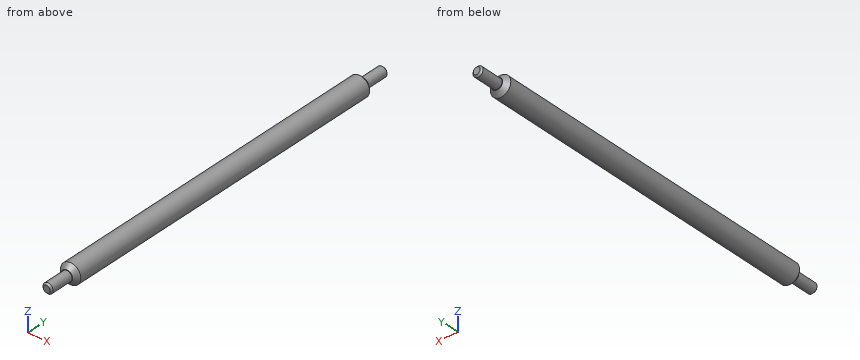
```python
from build123d import *

# Parameters (mm, degrees)
FASE1_SIZE = 2.2
FASE2_SIZE = 0.8


with BuildPart() as part:
    # Skizze1 → Rotation1 (revolve)
    with BuildSketch(Plane.XY, mode=Mode.PRIVATE) as rotation1_sk:
        Polygon((0, 0), (2.5, 0), (2.5, -12), (5, -12), (5, -188), (2.5, -188), (2.5, -200), (0, -200), align=None)
    revolve(rotation1_sk.sketch.rotate(Axis((0, 0, 0), (0, -1, 0)), 90), axis=Axis((0, 0, 0), (0, -1, 0)))

    # Fase1
    fase1_edges = [part.edges().sort_by_distance(p)[0] for p in [
        (0, -188, -5),
        (0, -12, -5),
    ]]
    chamfer(fase1_edges, length=FASE1_SIZE)

    # Fase2
    fase2_edges = [part.edges().sort_by_distance(p)[0] for p in [
        (0, -200, -2.5),
        (0, 0, -2.5),
    ]]
    chamfer(fase2_edges, length=FASE2_SIZE)


solid = part.part
```
Input: part model. Units: mm. Frame: model coordinates. Coordinates: 2 decimals unless noted, no trailing zeros. Loops run counter-clockwise (first coordinate to the right, second up) from the corner with the lowest first, then second, coordinate; pieces in that order, holes last. Notation, with made-up numbers: M -2.5,36.25 L 26.5,36.25 A17 cw 26.5,60.25 Z; hole C 59,47 d2. An arc over 180 degrees is marked long. Use a Markdown table: item, result. Add a question column.
1) Section C-C, the plane y = -34. Return the cut outline in (x, z), plus the area to 3 significant figures.
2) Pin query (flat end, axial travel): P1, Ø1, axis at x = 3.5, z = 0, coming from the +Y side; P2, Ø2, axis at y = -58.5, z = 1.5, coming from the -X side; P3, Ø1, axis at y = -144, z = 1.5, coming from the +X side. Return the tip coordinate at first contact, or that it passes through.
3) Section A-A, the plane x = 0. Return the cut outline in (y, z), plus the area to 3 significant figures.
4) Line query: L1, parallel to Y at x = 1.5, z = 2.25; L2, parallel to Z at x = 0.25, y = -31. Output: solid intervals per line, ascending. Write a range as from..to.
5) Section B-B, the plane z = 0. Return the cut outline in (x, y).
Answer below:
| question | item | result |
|---|---|---|
| 1 | outline | C 0,0 d10 |
| 1 | area | 78.5 mm2 |
| 2 | P1 | y = -12.2 |
| 2 | P2 | x = -4.97 |
| 2 | P3 | x = 4.9 |
| 3 | outline | M -200,-1.7 L -199.2,-2.5 L -188,-2.5 L -188,-2.8 L -185.8,-5 L -14.2,-5 L -12,-2.8 L -12,-2.5 L -0.8,-2.5 L 0,-1.7 L 0,1.7 L -0.8,2.5 L -12,2.5 L -12,2.8 L -14.2,5 L -185.8,5 L -188,2.8 L -188,2.5 L -199.2,2.5 L -200,1.7 Z |
| 3 | area | 1,870 mm2 |
| 4 | L1 | -188..-12 |
| 4 | L2 | -4.99..4.99 |
| 5 | outline | M -5,-185.8 L -2.8,-188 L -2.5,-188 L -2.5,-199.2 L -1.7,-200 L 1.7,-200 L 2.5,-199.2 L 2.5,-188 L 2.8,-188 L 5,-185.8 L 5,-14.2 L 2.8,-12 L 2.5,-12 L 2.5,-0.8 L 1.7,0 L -1.7,0 L -2.5,-0.8 L -2.5,-12 L -2.8,-12 L -5,-14.2 Z |
